Autodesk Fusion 360 part; units mm, degrees
sketch "スケッチ1" plane through (0, 0, 0) normal (0, 0, 1) x (1, 0, 0)
  arc A0 (21.7798, 234.5748) -> (9, 220.6281) centre (23, 220.6281) ccw
  line L0 (0, 250) -> (0, 0)
  line L1 (0, 0) -> (90, 0)
  line L2 (21.7798, 15.4252) -> (90, 9.4567)
  line L3 (9, 220.6281) -> (9, 29.3719)
  arc A1 (9, 29.3719) -> (21.7798, 15.4252) centre (23, 29.3719) ccw
  line L4 (90, 9.4567) -> (90, 0)
  line L5 (90, 240.5433) -> (21.7798, 234.5748)
  line L6 (0, 250) -> (90, 250)
  line L7 (90, 250) -> (90, 240.5433)
extrude "押し出し1" add sketch "スケッチ1" along normal blind 100
The listing builds one solid part. Answer for the finished solid, in the listing's coordinates (mm). A direction names the side the tool comes from. Give positions to 0.01 mm unless a question says otherwise; leave off trailing zeros. Order: outer loops, then holes, each group sorted by start corner. A loop starts at its lowest first (then second) coordinate and runs counter-clockwise, first axis right, second up. Notation, with made-up numbers: (-34.5, 12.25) -> (2.5, 12.25) arc R9 cw to (2.5, 24.25) -> close; hole circle Ø4 at (60, 83). An arc over 180 degrees is marked (long way). One line per item, written item: value.
1) Determine the mould class of faces 3 (the cylindrical face through (12.777, 19.807, 49.3)), 4 (the flat face through (90, 245, 49)), 5 (the flat face through (44, 250, 49)) for opening direction Y: pulls with the +Y half, pulls with the -Y half, needs draft (parallel to the pull), parting line crosses it, or undercut.
Reported:
face 3: undercut
face 4: needs draft
face 5: pulls with the +Y half
2) Find section D-D, the plane y = 194. Determine the outline of the cut face in (x, z).
Reported:
outline: (0, 0) -> (9, 0) -> (9, 100) -> (0, 100) -> close
3) A flat-ended cylindrical pin translates along its axis: P1, Ø10, axis at x = 18, y = 181, coming from the -Z side. Find the tip coordinate at first contact, or state that the pin passes through.
Reported:
P1: passes through
4) Find the intervals of material crossed by line 1 (X direction, y = 42, z = 64.5); line 2 (Y direction, x = 51, z = 15.5); line 3 (Y direction, x = 62, z = 22), in increasing order.
Reported:
line 1: x = 0 to 9
line 2: y = 0 to 12.87, 237.13 to 250
line 3: y = 0 to 11.91, 238.09 to 250
5) A tool of negligible diameter and unlimited length cuts with its end or side. For faces 1 (the flat face through (90, 5, 49)), 2 (the flat face through (9, 126, 49)), from which of +Z, -Z, +X, -X, +Y, -Y can it reach the whole face along a straight path? Write none if from no direction.
Reported:
face 1: +Z, -Z, +X, +Y, -Y
face 2: +Z, -Z, +X
6) Find section C-C, the plane x = 33. Determine the outline of the cut face in (y, z).
Reported:
outline: (0, 0) -> (14.44, 0) -> (14.44, 100) -> (0, 100) -> close; (235.56, 0) -> (250, 0) -> (250, 100) -> (235.56, 100) -> close
7) Find section B-B, the plane z = 55. Determine the outline of the cut face in (x, y).
Reported:
outline: (0, 0) -> (90, 0) -> (90, 9.46) -> (21.78, 15.43) arc R14 cw to (9, 29.37) -> (9, 220.63) arc R14 cw to (21.78, 234.57) -> (90, 240.54) -> (90, 250) -> (0, 250) -> close
8) Find section A-A, the plane x = 19. Determine the outline of the cut face in (y, z), plus the area to 3 significant figures.
Reported:
outline: (0, 0) -> (15.96, 0) -> (15.96, 100) -> (0, 100) -> close; (234.04, 0) -> (250, 0) -> (250, 100) -> (234.04, 100) -> close
area: 3,190 mm^2
